Build history of the part. All positions in model axes, mm. A direction names the side the tool comes from. Round coordinates to 2 decimals unless told otherwise and drop trailing zeros. Write each loop counter-clockwise with the first axis right and the second up, starting at its lowest first coordinate (ties: lowest second). Pieces come first, ordered by that corner, then holes.
1) Saw through at D-D (z = 7.25). Write the cut outline in (x, y), plus the area to 3 significant figures.
2) Which spindle directions (+Z, -Z, +X, -X, +Y, -Y) get a long thin tool onto all of the face, cutting with end or side? Do faces 1 (the flat face through (-13, 8, 4.953)), 2 (the cylindrical face through (-18.09, 5.95, 6.42)). Say none if no direction does.
3) Saw through at B-B (x = -6). Write the cut outline in (y, z).
4) Saw through at A-A (z = 5.5). Write the cut outline in (x, y).
5) Flat gauge pins, fed straight in: pin 1 (4 mm diameter, centred on x = -13, z = 3.5, fed in from +Y); pin 2 (2 mm diameter, centred on x = -12, y = 4.5, fed in from +Z); pin 3 (4 mm diameter, centred on x = -11.19, y = 3.09, fed in from +Z); pin 4 (4 mm diameter, centred on x = -9, z = 0, fed in from -Y). Where does each tip first touch, or does it go through?
6) Saw through at C-C (y = 8.25). Write the cut outline in (x, z), plus the area to 3 significant figures.
7) Wall check: probe 1 along Y at (x, z) = (-12.5, 1.5); probe 2 along X at (y, z) = (3.25, -0.25); probe 3 along Y at (x, z) = (-9.25, 6.5). Give the ranges that are in metal, low to high.
8) Pull direction Y, two halves, no side cores. Call faces 3 (the cylindrical face through (-8.644, 3.198, 1.77)), 4 (the cylindrical face through (-6.494, 4.566, 2.442)), 5 (the flat face through (-16, 3, 7.938)): +Y half, -Y half, draft (parallel to the pull), parting line (faces both ways), or undercut.
from build123d import *

# Parameters (mm, degrees)
SKETCH1_R                         = 4.9276
BOSS_EXTRUDE1_DEPTH               = 7.9375
SKETCH4_R                         = 4.9276
BOSS_EXTRUDE2_DEPTH               = 3.175
BOSS_EXTRUDE2_TAPER               = 45
F_1_4_20_TAPPED_HOLE1_D           = 5.1054
F_1_4_20_TAPPED_HOLE1_DEPTH       = 16.51
F_1_4_20_TAPPED_HOLE1_CSINK_D     = 8.9154
F_1_4_20_TAPPED_HOLE1_CSINK_ANGLE = 90
F_1_4_20_TAPPED_HOLE1_TIP         = 1.533816902
SKETCH5_W                         = 2.54
SKETCH5_H                         = 2.9845


with BuildPart() as part:
    # Sketch1 → Boss-Extrude1 (new body)
    with BuildSketch(Plane.XY):
        with Locations((-11.193990041, 3.085910768)):
            Circle(SKETCH1_R)
    extrude(amount=BOSS_EXTRUDE1_DEPTH)

    # Sketch4 → Boss-Extrude2 (add)
    with BuildSketch(Plane(origin=(0, 0, 0), x_dir=(-1, 0, 0), z_dir=(0, 0, -1))):
        with Locations((11.193990041, 3.085910768)):
            Circle(SKETCH4_R)
    extrude(amount=BOSS_EXTRUDE2_DEPTH, taper=BOSS_EXTRUDE2_TAPER)

    # 1/4-20 Tapped Hole1
    with Locations(Plane.XY.offset(7.9375)):
        with Locations((-11.193990041, 3.085910768)):
            CounterSinkHole(F_1_4_20_TAPPED_HOLE1_D / 2, F_1_4_20_TAPPED_HOLE1_CSINK_D / 2, depth=F_1_4_20_TAPPED_HOLE1_DEPTH, counter_sink_angle=F_1_4_20_TAPPED_HOLE1_CSINK_ANGLE)
            with Locations((0, 0, -(F_1_4_20_TAPPED_HOLE1_DEPTH + F_1_4_20_TAPPED_HOLE1_TIP / 2))):  # 118° drill point
                Cone(0, F_1_4_20_TAPPED_HOLE1_D / 2, F_1_4_20_TAPPED_HOLE1_TIP, mode=Mode.SUBTRACT)

    # Sketch5 → Revolve1 (revolve)
    with BuildSketch(Plane(origin=(0, 3.085910768, 0), x_dir=(1, 0, 0), z_dir=(0, 1, 0))):
        with Locations((-17.391590041, -6.44525)):
            Rectangle(SKETCH5_W, SKETCH5_H)
    revolve(axis=Axis((-11.193990041, 3.085910768, -2.3749), (0, 0, 1)))


solid = part.part
Evaluation:
1. outline: circle Ø14.94 at (-11.19, 3.09); hole circle Ø7.54 at (-11.19, 3.09)
1. area: 131 mm2
2. face 1: -Z
2. face 2: +Z, -Z
3. outline: (-2.28, 4.95) - (8.45, 4.95) - (8.45, 7.94) - (-2.28, 7.94) - close
4. outline: circle Ø14.94 at (-11.19, 3.09); hole circle Ø5.11 at (-11.19, 3.09)
5. pin 1: stops at y = 10.54
5. pin 2: stops at z = 6.11
5. pin 3: passes through
5. pin 4: stops at y = -1.84
6. outline: (-16.59, 4.95) - (-5.8, 4.95) - (-5.8, 7.94) - (-16.59, 7.94) - close
6. area: 32.2 mm2
7. probe 1: y = -1.67 to 0.89, 5.28 to 7.84
7. probe 2: x = -15.87 to -13.74, -8.65 to -6.52
7. probe 3: y = -4.12 to 0.77, 5.4 to 10.3
8. face 3: undercut
8. face 4: parting line
8. face 5: draft
